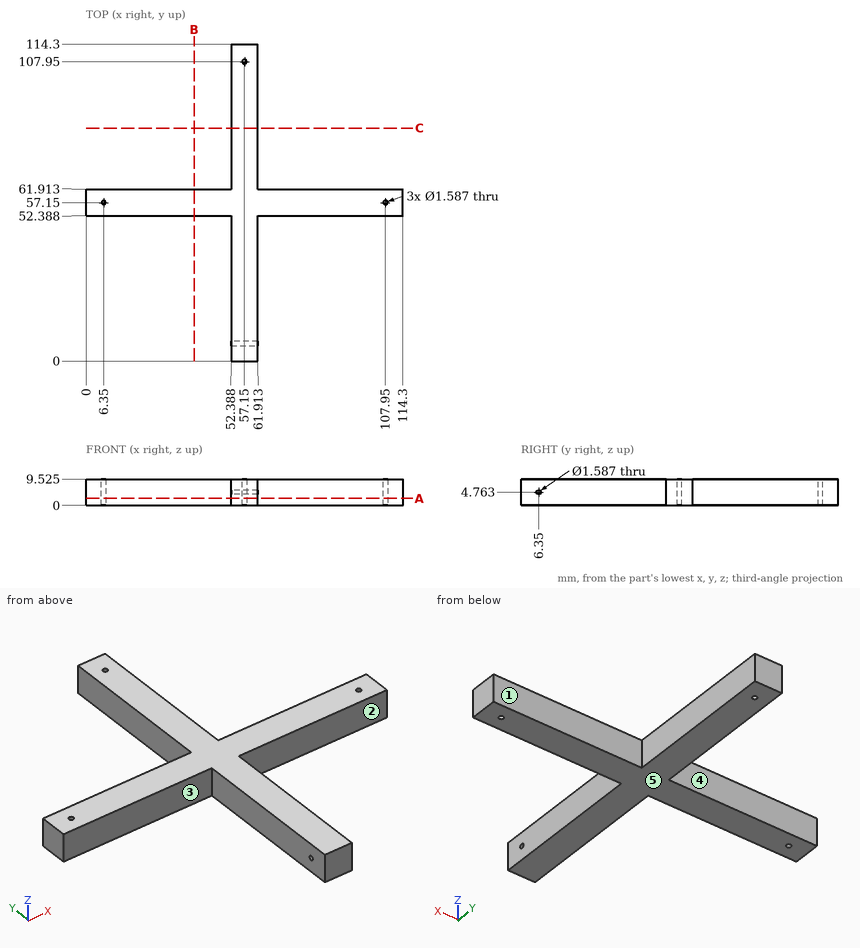
Input: dimensioned drawing with shaded views. Units: mm. Origin: part minimum x, y, z. A direction names the side the tool comes from. Give positions to 0.01 mm unless a question says otherwise; leave off trailing zeros. Order: outer loops, then holes, each group sorted by start corner. A loop starts at its lowest first (then second) coordinate and runs counter-clockwise, first axis right, second up.
(1) Contact query for flat-ended pins moving along their axis: P1, Ø1.4, axis at x = 6.35, y = 57.15, coming from the -Z side; P2, Ø3, axis at x = 77, z = 3.5, coming from the +Y side; P3, Ø5, axis at y = 33, z = 5, coming from the +X side; P4, Ø1, axis at y = 42.5, z = 7.5, coming from the -X side. Output: stop coordinate, or through.
(2) Section query B-B (x = 39). Return the cut outline in (y, z) (1 decimal).
(3) Section query A-A (z = 2.5). Return the cut outline in (x, y).
(4) Access query for the marked faces 1, 2, 3, 4 and 5. Directions: +Z, -Z, +X, -X, +Y, -Y. A direction counts if a zero-diameter tool reaches every point of the face in a straight line with its end or side. Return the directions, or none.
(5) Material intervals for line 1 along Y through (x, z) = (57.15, 7); line 2 along Y through (x, z) = (57.15, 4.75); line 3 along Z through (x, y) = (55, 6.35) (1 decimal), sorted ascending.
Outcome:
1. P1: passes through
1. P2: stops at y = 61.91
1. P3: stops at x = 61.91
1. P4: stops at x = 52.39
2. outline: (52.4, 0) - (61.9, 0) - (61.9, 9.5) - (52.4, 9.5) - close
3. outline: (0, 52.39) - (52.39, 52.39) - (52.39, 0) - (61.91, 0) - (61.91, 52.39) - (114.3, 52.39) - (114.3, 61.91) - (61.91, 61.91) - (61.91, 114.3) - (52.39, 114.3) - (52.39, 61.91) - (0, 61.91) - close; hole circle Ø1.59 at (6.35, 57.15); hole circle Ø1.59 at (57.15, 107.95); hole circle Ø1.59 at (107.95, 57.15)
4. face 1: +Z, -Z, +X, +Y
4. face 2: +Z, -Z, +X, -Y
4. face 3: +Z, -Z, -X, -Y
4. face 4: +Z, -Z, -X, +Y
4. face 5: -Z, +X, -X, +Y, -Y
5. line 1: y = 0 to 107.16, 108.74 to 114.3
5. line 2: y = 0 to 5.56, 7.14 to 107.16, 108.74 to 114.3
5. line 3: z = 0 to 4, 5.6 to 9.5
